Read the model definition and answer for the solid it produces. Units are mm, in the model's axes. A direction names the side the tool comes from. Round coordinates to 2 decimals unless told otherwise and drop trailing zeros. Order: outer loops, then holes, each group sorted by start corner. A loop starts at its lowest first (then second) coordinate and runs counter-clockwise, first axis right, second up. Notation, with made-up numbers: (55, 29.5) - (105, 29.5) arc R16 ccw to (105, 41.5) - close; hole circle Ø8 at (-10, -3.5). An arc over 180 degrees is marked (long way). Answer as a JSON object with one key per item and string values. Group by question number.
Q1. A cutting plane is placed at C-C on y = 0.8. Determine the outline of the cut face in (x, z), and give its area (3 significant figures).
Q2. The mould has two halves that part along X. Classify faces 1 (the cylindrical face through (19.55, 1.21, -0.43)), 2 (the flat face through (10, 2, -5)), 3 (the flat face through (10, 1, 0)), 4 (the conical face through (2.19, 0.25, -2.18)): pulls with the +X half, pulls with the -X half, needs draft (parallel to the pull), parting line crosses it, or undercut.
Q3. A tool of negligible diameter and unlimited length cuts with its end or side. For faces 5 (the flat face through (10, 2, -2)), 6 (the conical face through (2.18, 0.25, -4.81)), 7 (the flat face through (20, 1, -4)), from which of +Z, -Z, +X, -X, +Y, -Y can it reach the whole face along a straight path? Write none if from no direction.
Q4. A cutting plane is placed at A-A on z = -3.25. Determine the outline of the cut face in (x, y), and give its area (3 significant figures).
Q5. A cutting plane is placed at B-B on x = 15.75. Determine the outline of the cut face in (y, z).
Q6. Consider line 1 (Z direction, x = 8.25, y = 0.6); line 2 (X direction, y = 1.3, z = -3); line 3 (X direction, y = 0.7, z = -0.75). Determine where each line is inside the solid, lowest interval first.
```python
from build123d import *

# Parameters (mm, degrees)
SKETCH_1_W          = 20
SKETCH_1_H          = 6.1
EXTRUDE_1_DEPTH     = 3
SKETCH_2_W          = 16
SKETCH_2_H          = 3
CUT_EXTRUDE_1_DEPTH = 3
FILLET_1_R          = 1
FILLET_2_R          = 1.5
FILLET_3_R          = 1
CHAMFER_1_SIZE      = 0.4
FILLET_4_R          = 0.4
CHAMFER_2_SIZE      = 0.2


with BuildPart() as part:
    # 草图1 → 凸台-拉伸1 (new body)
    with BuildSketch(Plane(origin=(0, 0, 0), x_dir=(1, 0, 0), z_dir=(0, 1, 0))):
        with Locations((10, 3.05)):
            Rectangle(SKETCH_1_W, SKETCH_1_H)
    extrude(amount=EXTRUDE_1_DEPTH)

    # 草图2 → 切除-拉伸1 (cut)
    with BuildSketch(Plane(origin=(0, 3, 0), x_dir=(1, 0, 0), z_dir=(0, 1, 0))):
        with Locations((10, 3.5)):
            Rectangle(SKETCH_2_W, SKETCH_2_H)
    extrude(amount=-CUT_EXTRUDE_1_DEPTH, mode=Mode.SUBTRACT)

    # 圆角1
    fillet_1_edges = [part.edges().sort_by_distance(p)[0] for p in [
        (2, 1.5, -2),
        (2, 1.5, -5),
        (18, 1.5, -5),
        (18, 1.5, -2),
    ]]
    fillet(fillet_1_edges, radius=FILLET_1_R)

    # 圆角2
    fillet_2_edges = [part.edges().sort_by_distance(p)[0] for p in [
        (20, 1.5, 0),
        (0, 1.5, 0),
    ]]
    fillet(fillet_2_edges, radius=FILLET_2_R)

    # 圆角3
    fillet_3_edges = [part.edges().sort_by_distance(p)[0] for p in [
        (0, 3, -3.8),
        (10, 3, 0),
        (20, 3, -3.8),
        (19.560660172, 3, -0.439339828),
        (0.439339828, 3, -0.439339828),
    ]]
    fillet(fillet_3_edges, radius=FILLET_3_R)

    # 倒角1
    chamfer_1_edges = [part.edges().sort_by_distance(p)[0] for p in [
        (2, 0, -3.5),
        (10, 0, -5),
        (18, 0, -3.5),
        (10, 0, -2),
        (2.292893219, 0, -4.707106781),
        (17.707106781, 0, -4.707106781),
        (17.707106781, 0, -2.292893219),
        (2.292893219, 0, -2.292893219),
        (10, 0, 0),
        (20, 0, -3.8),
        (19.560660172, 0, -0.439339828),
        (0.439339828, 0, -0.439339828),
        (0, 0, -3.8),
    ]]
    chamfer(chamfer_1_edges, length=CHAMFER_1_SIZE)

    # 圆角4
    fillet_4_edges = [part.edges().sort_by_distance(p)[0] for p in [
        (2, 3, -3.5),
        (10, 3, -5),
        (18, 3, -3.5),
        (10, 3, -2),
        (2.292893219, 3, -4.707106781),
        (17.707106781, 3, -4.707106781),
        (17.707106781, 3, -2.292893219),
        (2.292893219, 3, -2.292893219),
    ]]
    fillet(fillet_4_edges, radius=FILLET_4_R)

    # 倒角2
    chamfer_2_edges = [part.edges().sort_by_distance(p)[0] for p in [
        (19.8, 0.2, -6.1),
        (0.2, 0.2, -6.1),
        (10, 3, -6.1),
        (0, 1.2, -6.1),
        (20, 1.2, -6.1),
        (19.707106781, 2.707106781, -6.1),
        (0.292893219, 2.707106781, -6.1),
        (10, 0, -6.1),
    ]]
    chamfer(chamfer_2_edges, length=CHAMFER_2_SIZE)


solid = part.part
```
Result set:
{
 "1": {"outline": "(0, -5.9) - (0.2, -6.1) - (19.8, -6.1) - (20, -5.9) - (20, -1.5) arc R1.5 ccw to (18.5, 0) - (1.5, 0) arc R1.5 ccw to (0, -1.5) - close; hole (2, -4) arc R1 ccw to (3, -5) - (17, -5) arc R1 ccw to (18, -4) - (18, -3) arc R1 ccw to (17, -2) - (3, -2) arc R1 ccw to (2, -3) - close", "area": "73.9 mm²"},
 "2": {"face 1": "pulls with the +X half", "face 2": "undercut", "face 3": "needs draft", "face 4": "undercut"},
 "3": {"face 5": "+Y, -Y", "face 6": "-Y", "face 7": "+Z, -Z, +X, +Y, -Y"},
 "4": {"outline": "(0, 0.4) - (0.4, 0) - (1.6, 0) - (2, 0.4) - (2, 2.6) arc R0.4 ccw to (1.6, 3) - (1, 3) arc R1 ccw to (0, 2) - close; (18, 0.4) - (18.4, 0) - (19.6, 0) - (20, 0.4) - (20, 2) arc R1 ccw to (19, 3) - (18.4, 3) arc R0.4 ccw to (18, 2.6) - close", "area": "11.2 mm²"},
 "5": {"outline": "(0, -5.9) - (0.2, -6.1) - (2.8, -6.1) - (3, -5.9) - (3, -5.4) arc R0.4 ccw to (2.6, -5) - (0.4, -5) - (0, -5.4) - close; (0, -1.6) - (0.4, -2) - (2.6, -2) arc R0.4 ccw to (3, -1.6) - (3, -1) arc R1 ccw to (2, 0) - (0.4, 0) - (0, -0.4) - close"},
 "6": {"line 1": "z = -6.1 to -5, -2 to 0", "line 2": "x = 0 to 2, 18 to 20", "line 3": "x = 0.2 to 19.8"}
}
